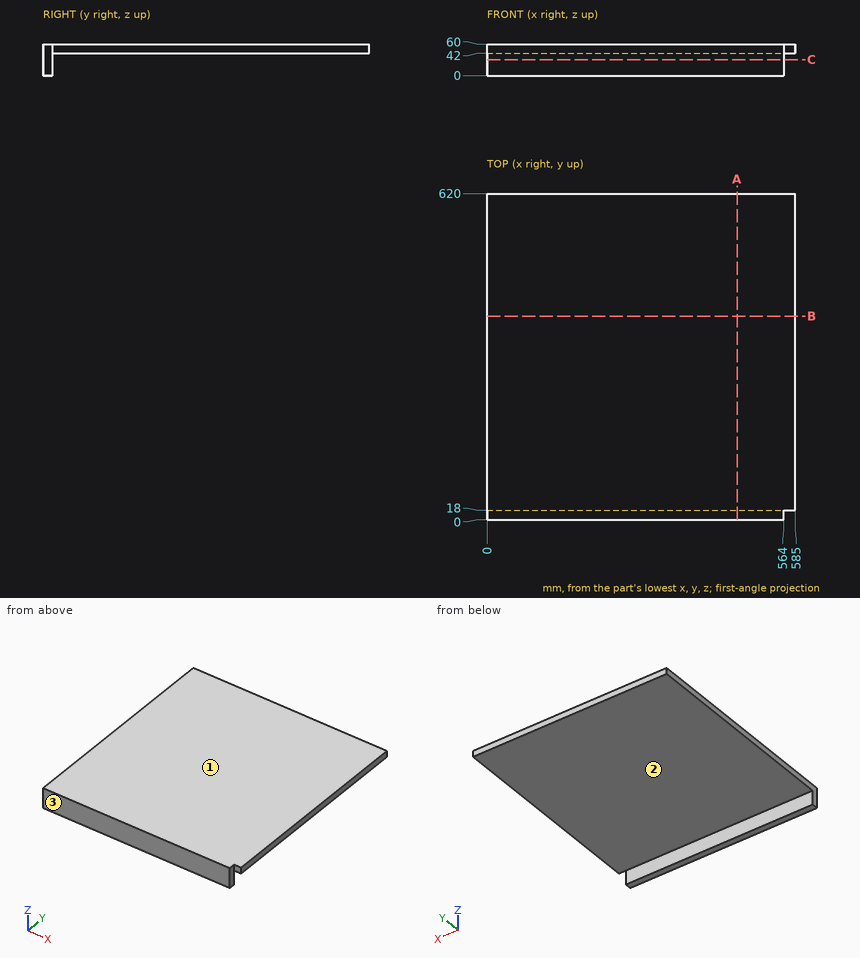
Design review of the part shown in the three views and the two pictorial views. Dimensions are in mm from the part's minimum x, y and z. Round coordinates to 2 decimals unless told otherwise and drop trailing zeros. Loops run counter-clockwise (first coordinate to the right, second up) from the corner with the lowest first, then second, coordinate; pieces in that order, holes last. Notation, with made-up numbers: M 46.5,49.25 L 83.5,49.25 A21 ccw 83.5,66.25 Z; hole C -1.5,12.5 d9. An arc over 180 degrees is marked long. Answer as a JSON object with one key per item and string values.
Item 1: We need section A-A on x = 475. Give the boundary of the cut face in (y, z).
Answer sheet:
{"outline": "M 0,0 L 18,0 L 18,42 L 620,42 L 620,60 L 0,60 Z"}
Item 2: We need section C-C on z = 30.5. Give the boundary of the cut face in (x, y).
Answer sheet:
{"outline": "M 0,0 L 564,0 L 564,18 L 0,18 Z"}
Item 3: We need section B-B on y = 387. Give the boundary of the cut face in (x, z).
Answer sheet:
{"outline": "M 0,42 L 585,42 L 585,60 L 0,60 Z"}
Item 4: Clearance check with flat-ended pins moving along their axes: P1, Ø5, axis at x = 377, y = 537, coming from the -Z side; P2, Ø10, axis at x = 188.5, z = 20.5, coming from the +Y side; P3, Ø14.5, axis at y = 10.5, z = 27, coming from the +X side; P4, Ø4, axis at x = 424, z = 10.5, coming from the -Y side. State where each tip first meets the part, or that it passes through.
Answer sheet:
{"P1": "stops at z = 42", "P2": "stops at y = 18", "P3": "stops at x = 564", "P4": "stops at y = 0"}
Item 5: The part is to be moulded in two halves that separate along Z. For the marked faces 1, 2 and 3, say which applies: pulls with the +Z half, pulls with the -Z half, needs draft (parallel to the pull), parting line crosses it, or undercut.
Answer sheet:
{"face 1": "pulls with the +Z half", "face 2": "pulls with the -Z half", "face 3": "needs draft"}
Item 6: Wall thickness on L1, parallel to Z at x = 69, y = 528.5; L2, parallel to Y at x = 313, z = 18: over which ranges is each line inside the solid? List them lowest first. Write a range as from..to.
Answer sheet:
{"L1": "z = 42..60", "L2": "y = 0..18"}
